The model under review builds one solid part; all positions refer to its coordinate system, in mm. Face numbers are marked on the shaded views. A direction names the side the tool comes from. Give positions to 0.01 mm unless a question says otherwise; leave off trailing zeros. Loops run counter-clockwise (first coordinate to the right, second up) from the corner with the lowest first, then second, coordinate; pieces in that order, holes last. Notation, with made-up numbers: M 35,75 L 70,75 A20 cw 70,90 Z; hole C 38.25,74 d11. An arc over 180 degrees is marked long. Return JSON: item names as keys, results as strings.
```python
from build123d import *

# Parameters (mm, degrees)
SKETCH1_R                  = 9.5
SKETCH1_R_2                = 2.15
BASE_FLANGE1_DEPTH         = 9.5
SKETCHED_START             = -98.25
SKETCHED_BEND1_OUTLINE_W   = 40
SKETCHED_BEND1_OUTLINE_H   = 9.5
SKETCHED_BEND1_DEPTH       = 51.5
SKETCHED_START_2           = -45.24247
SKETCHED_BEND1_2_OUTLINE_W = 40
SKETCHED_BEND1_2_OUTLINE_H = 56.113939487
SKETCHED_BEND1_2_OUTLINE_R = 2.15
SKETCHED_BEND1_2_DEPTH     = 7.99247
SKETCHED_START_3           = -46.75
SKETCHED_BEND1_3_OUTLINE_W = 40
SKETCHED_BEND1_3_OUTLINE_H = 56.113939487
SKETCHED_BEND1_3_OUTLINE_R = 2.15
SKETCHED_BEND1_3_DEPTH     = 15.5
SKETCHED_START_4           = 150
SKETCHED_BEND1_4_DEPTH     = 40


with BuildPart() as part:
    # Base-Flange1: sheet metal written as solids
    # Sketch1 → Base-Flange1 (new body)
    with BuildSketch(Plane(origin=(0, 0, 0), x_dir=(1, 0, 0), z_dir=(0, 1, 0))):
        with BuildLine():
            Line((0, -105), (0, -10))
            ThreePointArc((0, -10), (2.928932188, -2.928932188), (10, 0))
            Line((10, 0), (150, 0))
            Line((150, 0), (150, 98.25))
            Line((150, 98.25), (190, 98.25))
            Line((190, 98.25), (190, 0))
            ThreePointArc((190, 0), (229.599557186, -62.912629471), (176.5615547, -115))
            Line((176.5615547, -115), (10, -115))
            ThreePointArc((10, -115), (2.928932188, -112.071067812), (0, -105))
        make_face()
        with Locations(Location((41, -27, 0), (0, 0, 270))):
            Circle(SKETCH1_R, mode=Mode.SUBTRACT)
        with Locations(Location((41, -88, 0), (0, 0, 270))):
            Circle(SKETCH1_R, mode=Mode.SUBTRACT)
        with Locations(Location((160, 88.25, 0), (0, 0, 270))):
            Circle(SKETCH1_R_2, mode=Mode.SUBTRACT)
        with Locations(Location((180, 88.25, 0), (0, 0, 270))):
            Circle(SKETCH1_R_2, mode=Mode.SUBTRACT)
        with Locations(Location((180, 68.25, 0), (0, 0, 270))):
            Circle(SKETCH1_R_2, mode=Mode.SUBTRACT)
        with Locations(Location((160, 68.25, 0), (0, 0, 270))):
            Circle(SKETCH1_R_2, mode=Mode.SUBTRACT)
        with Locations(Location((75, -56.035702904, 0), (0, 0, 270))):
            Circle(SKETCH1_R, mode=Mode.SUBTRACT)
        with Locations(Location((119, -56.035702904, 0), (0, 0, 270))):
            Circle(SKETCH1_R, mode=Mode.SUBTRACT)
        with Locations(Location((97, -36, 0), (0, 0, 270))):
            Circle(SKETCH1_R, mode=Mode.SUBTRACT)
        with Locations(Location((97, -79, 0), (0, 0, 270))):
            Circle(SKETCH1_R, mode=Mode.SUBTRACT)
        with Locations(Location((155, -27, 0), (0, 0, 270))):
            Circle(SKETCH1_R, mode=Mode.SUBTRACT)
        with Locations(Location((182, -56.035702904, 0), (0, 0, 270))):
            Circle(SKETCH1_R, mode=Mode.SUBTRACT)
        with Locations(Location((155, -88, 0), (0, 0, 270))):
            Circle(SKETCH1_R, mode=Mode.SUBTRACT)
    extrude(amount=BASE_FLANGE1_DEPTH)

    # Sketched Bend1: read off the stored shape, not the designer's step
    # Sketched Bend1 outline → Sketched Bend1 (cut)
    with BuildSketch(Plane.XY.offset(SKETCHED_START)):
        with Locations((170, 4.75)):
            Rectangle(SKETCHED_BEND1_OUTLINE_W, SKETCHED_BEND1_OUTLINE_H)
    extrude(amount=SKETCHED_BEND1_DEPTH, mode=Mode.SUBTRACT)

    # Sketched Bend1 2 outline → Sketched Bend1 2 (add)
    with BuildSketch(Plane.XY.offset(SKETCHED_START_2)):
        with Locations((170, 37.556969744)):
            Rectangle(SKETCHED_BEND1_2_OUTLINE_W, SKETCHED_BEND1_2_OUTLINE_H)
        with Locations((160, 35.613939487)):
            Circle(SKETCHED_BEND1_2_OUTLINE_R, mode=Mode.SUBTRACT)
        with Locations((160, 55.613939487)):
            Circle(SKETCHED_BEND1_2_OUTLINE_R, mode=Mode.SUBTRACT)
        with Locations((180, 35.613939487)):
            Circle(SKETCHED_BEND1_2_OUTLINE_R, mode=Mode.SUBTRACT)
        with Locations((180, 55.613939487)):
            Circle(SKETCHED_BEND1_2_OUTLINE_R, mode=Mode.SUBTRACT)
    extrude(amount=SKETCHED_BEND1_2_DEPTH)

    # Sketched Bend1 3 outline → Sketched Bend1 3 (add)
    with BuildSketch(Plane.XY.offset(SKETCHED_START_3)):
        with Locations((170, 37.556969744)):
            Rectangle(SKETCHED_BEND1_3_OUTLINE_W, SKETCHED_BEND1_3_OUTLINE_H)
        with Locations((160, 35.613939487)):
            Circle(SKETCHED_BEND1_3_OUTLINE_R, mode=Mode.SUBTRACT)
        with Locations((180, 35.613939487)):
            Circle(SKETCHED_BEND1_3_OUTLINE_R, mode=Mode.SUBTRACT)
        with Locations((160, 55.613939487)):
            Circle(SKETCHED_BEND1_3_OUTLINE_R, mode=Mode.SUBTRACT)
        with Locations((180, 55.613939487)):
            Circle(SKETCHED_BEND1_3_OUTLINE_R, mode=Mode.SUBTRACT)
    extrude(amount=SKETCHED_BEND1_3_DEPTH)

    # Sketched Bend1 4 outline → Sketched Bend1 4 (cut)
    with BuildSketch(Plane.YZ.offset(SKETCHED_START_4)):
        with BuildLine():
            ThreePointArc((9.5, -31.25), (11.257359313, -35.492640687), (15.5, -37.25))
            Line((15.5, -37.25), (65.613939487, -37.25))
            Line((65.613939487, -37.25), (65.613939487, -31.25))
            Line((65.613939487, -31.25), (9.5, -31.25))
        make_face()
        with BuildLine():
            Line((0, -46.75), (15.5, -46.75))
            ThreePointArc((15.5, -46.75), (4.539844892, -42.210155108), (0, -31.25))
            Line((0, -31.25), (0, -46.75))
        make_face()
    extrude(amount=SKETCHED_BEND1_4_DEPTH, mode=Mode.SUBTRACT)


solid = part.part
```
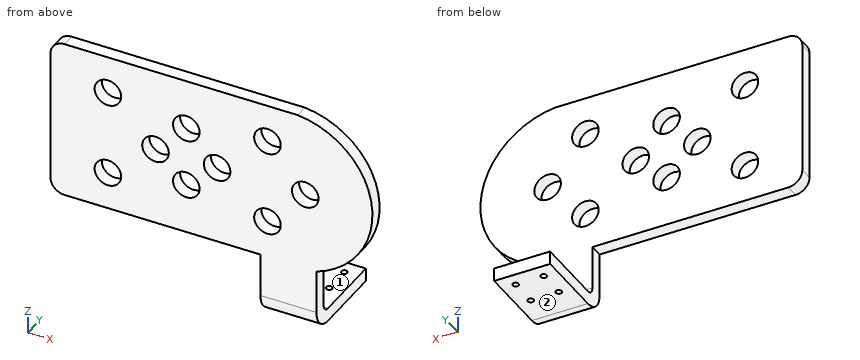
1) Insertion check: pin 1 (6 mm diameter, centred on x = 166, z = -4, fed in from +Y). The pin has a flat end and moves straight along its axis. Give the tip position at first contact, or say it passes through.
From the geometry:
{"pin 1": "y = 9.5"}
2) Consider section D-D on y = 27.5. Write out the cut boundary in (x, z).
From the geometry:
{"outline": "M 150,-46.75 L 190,-46.75 L 190,-37.25 L 150,-37.25 Z"}
3) Wall thickness on L1, parallel to Y at x = 192.5, z = 77; L2, parallel to Y at x = 160, z = -40; L3, parallel to Z at x = 151, y = 49: over which ranges is each line inside the solid? List them lowest first. Write a range as from..to.
From the geometry:
{"L1": "0..9.5", "L2": "2.71..33.46, 37.76..53.46, 57.76..65.61", "L3": "-46.75..-37.25"}
4) Tool access review of the marked faces 1 and 2: name each direction out of +Z, -Z, +X, -X, +Y, -Y from which nothing blocks a thin tool from reaching the whole face with its end or side.
From the geometry:
{"face 1": "+Z, +X, -X, +Y", "face 2": "-Z, +X, -X, +Y, -Y"}
5) Consider section B-B on z = 53.5. Write out the cut boundary in (x, y), then the cut area to 3 significant figures.
From the geometry:
{"outline": "M 0,0 L 65.84,0 L 65.84,9.5 L 0,9.5 Z; M 84.16,0 L 109.84,0 L 109.84,9.5 L 84.16,9.5 Z; M 128.16,0 L 172.84,0 L 172.84,9.5 L 128.16,9.5 Z; M 191.16,0 L 229.95,0 L 229.95,9.5 L 191.16,9.5 Z", "area": "1,660 mm²"}
6) Consider section A-A on x = 41. Write out the cut boundary in (y, z).
From the geometry:
{"outline": "M 0,0 L 9.5,0 L 9.5,17.5 L 0,17.5 Z; M 0,36.5 L 9.5,36.5 L 9.5,78.5 L 0,78.5 Z; M 0,97.5 L 9.5,97.5 L 9.5,115 L 0,115 Z"}
7) Consider section C-C on z = 74.5. Write out the cut boundary in (x, y).
From the geometry:
{"outline": "M 0,0 L 88.63,0 L 88.63,9.5 L 0,9.5 Z; M 105.37,0 L 227.05,0 L 227.05,9.5 L 105.37,9.5 Z"}
